CAD build for the part. Positions are in the model's coordinates, mm. A direction names the side the tool comes from. Give positions to 0.01 mm unless a question says otherwise; leave off trailing zeros. Write each loop counter-clockwise with the first axis right and the second up, starting at its lowest first coordinate (ties: lowest second). Pieces come first, ordered by that corner, then holes. Notation, with made-up numbers: (-25, 36.25) - (-11, 36.25) arc R32 ccw to (-11, 73.25) - close; hole circle Ø8 at (-12.75, 74). An arc over 180 degrees is marked (long way). Put each result on its own line as item: value. Start each with the question number.
1. Cut at B-B on y = 19.75. Give the number of separate pieces and of enclosed holes in the cut face, and give its area (3 significant figures).
2. Tool access for faces 1 (the cylindrical face through (22.08, 18.37, 99.43)), 2 (the cylindrical face through (-67.01, 12.49, 89.71)): list every direction of +Z, -Z, +X, -X, +Y, -Y with a clear straight run to the whole face (end or side of a thin tool).
3. Wall check: line 1 (X direction, y = 14, z = 0); line 2 (Z direction, x = -112, y = 22.5); line 3 (X direction, y = 21.75, z = 47). Give the ranges that are in metal, low to high.
4. Drop flat-ended pins along their axis: pin 1 (1 mm diameter, centred on x = 34.5, y = 9, fed in from +Z); pin 2 (5 mm diameter, centred on x = -65, y = 13, fed in from +Z); pin 3 (3 mm diameter, centred on x = 15, y = 13, fed in from +Z). Give the stop position or say it passes through.
5. Cut at A-A on x = 0. List the corners of the cut face in (y, z) (3 decimals), and give its area (3 significant figures).
from build123d import *

# Parameters (mm, degrees)
SKETCH1_R                    = 126.619
SKETCH1_R_2                  = 99.2124
BOSS_EXTRUDE1_DEPTH          = 24.638
SKETCH2_R                    = 101.854
CUT_EXTRUDE1_DEPTH           = 11.938
CHAMFER1_SIZE                = 0.762
SKETCH3_R                    = 4.2164
CUT_EXTRUDE2_DEPTH           = 25.638
CHAMFER2_SIZE                = 0.381
CIRPATTERN1_COUNT            = 24
CHAMFER2_OF_CIRPATTERN1_SIZE = 0.381
CUT_EXTRUDE3_DEPTH           = 0.79375


with BuildPart() as part:
    # Sketch1 → Boss-Extrude1 (new body)
    with BuildSketch(Plane(origin=(0, 0, 0), x_dir=(1, 0, 0), z_dir=(0, 1, 0))):
        Circle(SKETCH1_R)
        Circle(SKETCH1_R_2, mode=Mode.SUBTRACT)
    extrude(amount=BOSS_EXTRUDE1_DEPTH)

    # Sketch2 → Cut-Extrude1 (cut)
    with BuildSketch(Plane(origin=(0, 24.638, 0), x_dir=(-1, 0, 0), z_dir=(0, -1, 0))):
        Circle(SKETCH2_R)
    extrude(amount=CUT_EXTRUDE1_DEPTH, mode=Mode.SUBTRACT)

    # Chamfer1
    chamfer1_edges = [part.edges().sort_by_distance(p)[0] for p in [
        (101.854, 24.638, 0),
        (-126.619, 0, 0),
        (-126.619, 24.638, 0),
    ]]
    chamfer(chamfer1_edges, length=CHAMFER1_SIZE)

    # Sketch4 → Cut-Revolve1 (revolve, cut)
    with BuildSketch(Plane.XY):
        Polygon((-111.125, 0), (-111.125, 1.6256), (-108.458, 0.6604), (-108.458, 1.27), (0, 1.27), (0, 0), align=None)
    revolve(axis=Axis((0, 24.638, 0), (0, -1, 0)), mode=Mode.SUBTRACT)

    # Sketch3 → Cut-Extrude2 (cut, through all)
    with BuildSketch(Plane(origin=(0, 24.638, 0), x_dir=(1, 0, 0), z_dir=(0, 1, 0))):
        with Locations((-15.131327149, 114.933840422)):
            Circle(SKETCH3_R)
    cut_extrude2 = extrude(amount=-CUT_EXTRUDE2_DEPTH, mode=Mode.SUBTRACT)

    # Chamfer2
    chamfer2_edges = [part.edges().sort_by_distance(p)[0] for p in [
        (-19.347727149, 0, -114.933840422),
        (-19.347727149, 24.638, -114.933840422),
    ]]
    chamfer(chamfer2_edges, length=CHAMFER2_SIZE)

    # CirPattern1: Cut-Extrude2 ×24 about axis
    cirpattern1_axis = Axis((0, 0, 0), (0, 1, 0))
    for i in range(1, CIRPATTERN1_COUNT):
        add(cut_extrude2.rotate(cirpattern1_axis, i * 360 / CIRPATTERN1_COUNT), mode=Mode.SUBTRACT)

    # Chamfer2 of CirPattern1
    chamfer2_of_cirpattern1_edges = [part.edges().sort_by_distance(p)[0] for p in [
        (-48.435536161, 0, -106.010004512),
        (-48.435536161, 24.638, -106.010004512),
        (-74.222543427, 0, -89.861761985),
        (-74.222543427, 24.638, -89.861761985),
        (-94.951407017, 0, -67.589588882),
        (-94.951407017, 24.638, -67.589588882),
        (-109.209489134, 0, -40.711296994),
        (-109.209489134, 24.638, -40.711296994),
        (-116.025125043, 0, -11.058597495),
        (-116.025125043, 24.638, -11.058597495),
        (-114.933840422, 0, 19.347727149),
        (-114.933840422, 24.638, 19.347727149),
        (-106.010004512, 0, 48.435536161),
        (-106.010004512, 24.638, 48.435536161),
        (-89.861761985, 0, 74.222543427),
        (-89.861761985, 24.638, 74.222543427),
        (-67.589588882, 0, 94.951407017),
        (-67.589588882, 24.638, 94.951407017),
        (-40.711296994, 0, 109.209489134),
        (-40.711296994, 24.638, 109.209489134),
        (-11.058597495, 0, 116.025125043),
        (-11.058597495, 24.638, 116.025125043),
        (19.347727149, 0, 114.933840422),
        (19.347727149, 24.638, 114.933840422),
        (48.435536161, 0, 106.010004512),
        (48.435536161, 24.638, 106.010004512),
        (74.222543427, 0, 89.861761985),
        (74.222543427, 24.638, 89.861761985),
        (94.951407017, 0, 67.589588882),
        (94.951407017, 24.638, 67.589588882),
        (109.209489134, 0, 40.711296994),
        (109.209489134, 24.638, 40.711296994),
        (116.025125043, 0, 11.058597495),
        (116.025125043, 24.638, 11.058597495),
        (114.933840422, 0, -19.347727149),
        (114.933840422, 24.638, -19.347727149),
        (106.010004512, 0, -48.435536161),
        (106.010004512, 24.638, -48.435536161),
        (89.861761985, 0, -74.222543427),
        (89.861761985, 24.638, -74.222543427),
        (67.589588882, 0, -94.951407017),
        (67.589588882, 24.638, -94.951407017),
        (40.711296994, 0, -109.209489134),
        (40.711296994, 24.638, -109.209489134),
        (11.058597495, 0, -116.025125043),
        (11.058597495, 24.638, -116.025125043),
    ]]
    chamfer(chamfer2_of_cirpattern1_edges, length=CHAMFER2_OF_CIRPATTERN1_SIZE)

    # Sketch5 → Cut-Extrude3 (cut, symmetric)
    with BuildSketch(Plane.XY):
        Polygon((-109.62454103, 0.887787398), (-126.619, 1.778429253), (-126.619, -4.857391352), (-109.62454103, -4.857391352), align=None)
        Polygon((109.62454103, 0.887787398), (109.62454103, -4.857391352), (126.619, -4.857391352), (126.619, 1.778429253), align=None)
    extrude(amount=CUT_EXTRUDE3_DEPTH, both=True, mode=Mode.SUBTRACT)


solid = part.part
Report:
1. separate pieces: 1
1. enclosed holes: 25
1. area: 16,400 mm²
2. face 1: +Y
2. face 2: +Y, -Y
3. line 1: x = -126.62 to -101.85, 101.85 to 126.62
3. line 2: z = -59.06 to -18.16, -12.1 to 12.1, 18.16 to 59.06
3. line 3: x = -117.57 to -110.39, -103.81 to -90.36, 90.36 to 103.81, 110.39 to 117.57
4. pin 1: stops at z = 121.97
4. pin 2: stops at z = 110.12
4. pin 3: stops at z = 125.9
5. outline: (0, -125.857) - (0.762, -126.619) - (23.876, -126.619) - (24.638, -125.857) - (24.638, -102.616) - (23.876, -101.854) - (12.7, -101.854) - (12.7, -99.212) - (1.27, -99.212) - (1.27, -108.458) - (0.66, -108.458) - (1.626, -111.125) - (0, -111.125) - close; (0, 111.125) - (1.626, 111.125) - (0.66, 108.458) - (1.27, 108.458) - (1.27, 99.212) - (12.7, 99.212) - (12.7, 101.854) - (23.876, 101.854) - (24.638, 102.616) - (24.638, 125.857) - (23.876, 126.619) - (0.762, 126.619) - (0, 125.857) - close
5. area: 1,260 mm²
